Geometry check sheet. Reference: the model listing, model coordinates, mm. A direction names the side the tool comes from. Give positions to 0.01 mm unless a question says otherwise; leave off trailing zeros. Order: outer loops, then holes, each group sorted by start corner. A loop starts at its lowest first (then second) coordinate and runs counter-clockwise, first axis right, second up.
```python
from build123d import *

# Parameters (mm, degrees)
SKETCH_1_W                  = 32
SKETCH_1_H                  = 22
EXTRUDE_1_DEPTH             = 2.5
EXTRUDE_2_DEPTH             = 6
EXTRUDE_3_DEPTH             = 6
EXTRUDE_START               = -6
EXTRUDE_4_DEPTH             = 6
EXTRUDE_5_DEPTH             = 6
HOLE_WIZARD_3_4_3_4_1_D     = 3.4
HOLE_WIZARD_3_4_3_4_1_DEPTH = 6
HOLE_WIZARD_3_4_3_4_2_D     = 3.4
HOLE_WIZARD_3_4_3_4_2_DEPTH = 6
HOLE_WIZARD_3_4_3_4_3_D     = 3.4
HOLE_WIZARD_3_4_3_4_4_D     = 3.4
HOLE_WIZARD_3_4_3_4_4_DEPTH = 22
HOLE_WIZARD_3_2_3_2_1_D     = 3.2
HOLE_WIZARD_10_5_10_5_1_D   = 10.5
EXTRUDE_START_2             = 2
SKETCH_18_R                 = 1.6
SKETCH_18_R_2               = 5.25
EXTRUDE_7_DEPTH             = 2
RIB_1_REACH                 = 43.485
SKETCH_20_WALL_W            = 88.17143617
SKETCH_20_WALL_H            = 32
RIB_2_REACH                 = 43.485
SKETCH_22_WALL_W            = 88.17143617
SKETCH_22_WALL_H            = 32


with BuildPart() as part:
    # 草图1 → 凸台-拉伸1 (new body)
    with BuildSketch(Plane(origin=(0, 0, 0), x_dir=(-1, 0, 0), z_dir=(0, 0, -1))):
        Rectangle(SKETCH_1_W, SKETCH_1_H)
    extrude(amount=-EXTRUDE_1_DEPTH)

    # 草图2 → 凸台-拉伸2 (add)
    with BuildSketch(Plane(origin=(0, 11, 0), x_dir=(1, 0, 0), z_dir=(0, 1, 0))):
        with BuildLine():
            Line((9, 5), (9, 1))
            ThreePointArc((9, 1), (8.707106781, 0.292893219), (8, 0))
            Line((8, 0), (16, 0))
            Line((16, 0), (16, 5))
            ThreePointArc((16, 5), (12.5, 8.5), (9, 5))
        make_face()
    extrude(amount=-EXTRUDE_2_DEPTH)

    # 草图3 → 凸台-拉伸3 (add)
    with BuildSketch(Plane(origin=(0, 11, 0), x_dir=(1, 0, 0), z_dir=(0, 1, 0))):
        with BuildLine():
            Line((-16, 0), (-8, 0))
            ThreePointArc((-8, 0), (-8.707106781, 0.292893219), (-9, 1))
            Line((-9, 1), (-9, 5))
            ThreePointArc((-9, 5), (-12.5, 8.5), (-16, 5))
            Line((-16, 5), (-16, 0))
        make_face()
    extrude(amount=-EXTRUDE_3_DEPTH)

    # 草图4 → 凸台-拉伸4 (add)
    with BuildSketch(Plane.XZ.offset(11).offset(EXTRUDE_START)):
        with BuildLine():
            Line((-8, 0), (-16, 0))
            Line((-16, 0), (-16, -5))
            ThreePointArc((-16, -5), (-12.5, -8.5), (-9, -5))
            Line((-9, -5), (-9, -1))
            ThreePointArc((-9, -1), (-8.707106781, -0.292893219), (-8, 0))
        make_face()
    extrude(amount=EXTRUDE_4_DEPTH)

    # 草图5 → 凸台-拉伸5 (add)
    with BuildSketch(Plane.XZ.offset(11).offset(EXTRUDE_START)):
        with BuildLine():
            Line((16, -5), (16, 0))
            Line((16, 0), (8, 0))
            ThreePointArc((8, 0), (8.707106781, -0.292893219), (9, -1))
            Line((9, -1), (9, -5))
            ThreePointArc((9, -5), (12.5, -8.5), (16, -5))
        make_face()
    extrude(amount=EXTRUDE_5_DEPTH)

    # Ø3.4 (3.4) 直径孔1
    with Locations(Plane(origin=(0, -5, 0), x_dir=(1, 0, 0), z_dir=(0, 1, 0))):
        with Locations((-12.5, 5)):
            Hole(HOLE_WIZARD_3_4_3_4_1_D / 2, depth=HOLE_WIZARD_3_4_3_4_1_DEPTH)

    # Ø3.4 (3.4) 直径孔2
    with Locations(Plane(origin=(0, -11, 0), x_dir=(-1, 0, 0), z_dir=(0, -1, 0))):
        with Locations((-12.5, 5)):
            Hole(HOLE_WIZARD_3_4_3_4_2_D / 2, depth=HOLE_WIZARD_3_4_3_4_2_DEPTH)

    # Ø3.4 (3.4) 直径孔3 (through all)
    with Locations(Plane(origin=(0, 5, 0), x_dir=(-1, 0, 0), z_dir=(0, -1, 0))):
        with Locations((12.5, 5)):
            Hole(HOLE_WIZARD_3_4_3_4_3_D / 2)

    # Ø3.4 (3.4) 直径孔4
    with Locations(Plane(origin=(0, 11, 0), x_dir=(1, 0, 0), z_dir=(0, 1, 0))):
        with Locations((12.5, 5)):
            Hole(HOLE_WIZARD_3_4_3_4_4_D / 2, depth=HOLE_WIZARD_3_4_3_4_4_DEPTH)

    # Ø3.2 (3.2) 直径孔1 (through all)
    with Locations(Plane(origin=(0, 0, 0), x_dir=(-1, 0, 0), z_dir=(0, 0, -1))):
        with Locations((5.656854249, 5.656854249), (-5.656854249, 5.656854249), (-5.656854249, -5.656854249), (5.656854249, -5.656854249)):
            Hole(HOLE_WIZARD_3_2_3_2_1_D / 2)

    # Ø10.5 (10.5) 直径孔1 (through all)
    with Locations(Plane(origin=(0, 0, 0), x_dir=(-1, 0, 0), z_dir=(0, 0, -1))):
        with Locations((0, 0)):
            Hole(HOLE_WIZARD_10_5_10_5_1_D / 2)

    # 草图18 → 凸台-拉伸7 (add)
    with BuildSketch(Plane.XY.offset(2.5).offset(EXTRUDE_START_2)):
        Polygon((-16, 11), (-16, 13), (16, 13), (16, 11), (16, -11), (16, -13), (-16, -13), (-16, -11), align=None)
        with Locations(Location((-5.656854249, 5.656854249, 0), (0, 0, 180))):
            Circle(SKETCH_18_R, mode=Mode.SUBTRACT)
        with Locations(Location((5.656854249, 5.656854249, 0), (0, 0, 180))):
            Circle(SKETCH_18_R, mode=Mode.SUBTRACT)
        with Locations(Location((5.656854249, -5.656854249, 0), (0, 0, 180))):
            Circle(SKETCH_18_R, mode=Mode.SUBTRACT)
        with Locations(Location((-5.656854249, -5.656854249, 0), (0, 0, 180))):
            Circle(SKETCH_18_R, mode=Mode.SUBTRACT)
        with Locations(Location((0, 0, 0), (0, 0, 180))):
            Circle(SKETCH_18_R_2, mode=Mode.SUBTRACT)
    extrude(amount=-EXTRUDE_7_DEPTH)

    # 草图20 wall → 筋1 (add, up to next)
    with BuildSketch(Plane(origin=(-16, -12, 1.25), x_dir=(0, 0.624695047554, -0.780868809443), z_dir=(0, -0.780868809443, -0.624695047554)), mode=Mode.PRIVATE) as rib_1_sk1:
        with Locations((0, 16)):
            Rectangle(SKETCH_20_WALL_W, SKETCH_20_WALL_H)
    rib_1_tool1 = extrude(rib_1_sk1.sketch, amount=-RIB_1_REACH, mode=Mode.PRIVATE) - part.part
    add(rib_1_tool1.solids().sort_by_distance((-16, -12, 1.25))[0])

    # 草图22 wall → 筋2 (add, up to next)
    with BuildSketch(Plane(origin=(16, 12, 1.25), x_dir=(0, -0.624695047554, -0.780868809443), z_dir=(0, 0.780868809443, -0.624695047554)), mode=Mode.PRIVATE) as rib_2_sk1:
        with Locations((0, 16)):
            Rectangle(SKETCH_22_WALL_W, SKETCH_22_WALL_H)
    rib_2_tool1 = extrude(rib_2_sk1.sketch, amount=-RIB_2_REACH, mode=Mode.PRIVATE) - part.part
    add(rib_2_tool1.solids().sort_by_distance((16, 12, 1.25))[0])


solid = part.part
```
Q1. Access from +Z, -Z, +X, -X, +Y, -Y to the whole of each face (thin tool, end or side, straight path). Record for faces 1 (the face through (-9, 8, -3)), 2 (the face through (-12, -11, -3)), 3 (the face through (-11, 5, -3)), 4 (the face through (-11, 11, -3)), 5 (the face through (0, 13, 4)).
Q2. Cross-section at D-D, the plane y = 0. Record the boundary of the cut face in (x, z).
Q3. Cross-section at A-A, the plane x = 0. Record the boundary of the cut face in (y, z).
Q4. Cross-section at C-C, the plane x = 12.5. Record the boundary of the cut face in (y, z).
Q5. Cross-section at B-B, the plane y = -8. Record the boundary of the cut face in (x, z).
Q6. Thickness scan on L1, parallel to Y at x = -12, z = -0.5; L2, parallel to X at y = -7.5, z = -4; L3, parallel to Z at x = 12.5, y = -7.6. Record the ranges inside material, lowest first.
Q7. Gauge pin test, flat ends, axial feed: P1, Ø3, axis at y = 4, z = -7, coming from the +X side; P2, Ø2, axis at x = 0, y = -7, coming from the -Z side; P3, Ø6.5, axis at x = -12, z = -3, coming from the +Y side. Record the tip position at first contact, or that the pin passes through.
Q8. Release check for a two-part mould opening along Y. For faces 6 (the face through (12, -11, -3)), 7 (the face through (9, -8, -3)), 8 (the face through (12, -5, -3)) record: pulls with the +Y half, pulls with the -Y half, needs draft (parallel to the pull), parting line crosses it, or undercut.
Answers follow:
1. face 1: -Z, +Y, -Y
1. face 2: -Z, +X, -X, -Y
1. face 3: -Z, +X, -X
1. face 4: -Z, +X, -X, +Y
1. face 5: +Z, -Z, +X, -X, +Y
2. outline: (-16, 0) - (-5.25, 0) - (-5.25, 4.5) - (-16, 4.5) - close; (5.25, 0) - (16, 0) - (16, 4.5) - (5.25, 4.5) - close
3. outline: (-13, 2.5) - (-11, 0) - (-5.25, 0) - (-5.25, 4.5) - (-13, 4.5) - close; (5.25, 0) - (11, 0) - (13, 2.5) - (13, 4.5) - (5.25, 4.5) - close
4. outline: (-13, 2.5) - (-11, 0) - (-11, -3.3) - (-5, -3.3) - (-5, 0) - (5, 0) - (5, -3.3) - (11, -3.3) - (11, 0) - (13, 2.5) - (13, 4.5) - (-13, 4.5) - close; (-11, -8.5) - (-5, -8.5) - (-5, -6.7) - (-11, -6.7) - close; (5, -8.5) - (11, -8.5) - (11, -6.7) - (5, -6.7) - close
5. outline: (-16, -5) arc R3.5 ccw to (-9, -5) - (-9, -1) arc R1 cw to (-8, 0) - (8, 0) arc R1 cw to (9, -1) - (9, -5) arc R3.5 ccw to (16, -5) - (16, 4.5) - (-16, 4.5) - close; hole circle Ø3.4 at (-12.5, -5); hole circle Ø3.4 at (12.5, -5)
6. L1: y = -11 to -5, 5 to 11
6. L2: x = -16 to -13.87, -11.13 to -9, 9 to 11.13, 13.87 to 16
6. L3: z = -8.5 to -6.7, -3.3 to 4.5
7. P1: stops at x = 15.89
7. P2: stops at z = 0
7. P3: stops at y = 11.2
8. face 6: pulls with the -Y half
8. face 7: needs draft
8. face 8: undercut
